CAD build for the part. Positions are in the model's coordinates, mm. Face numbers are marked on the shaded views. A direction names the side the tool comes from. Coordinates: 2 decimals unless noted, no trailing zeros. Order: outer loops, then holes, each group sorted by start corner. A loop starts at its lowest first (then second) coordinate and runs counter-clockwise, first axis right, second up. Notation, with made-up numbers: M 30.25,6 L 46.25,6 A28 ccw 46.25,37 Z; hole C -18.5,11 d5. An arc over 180 degrees is marked long. Write item = value, one per line.
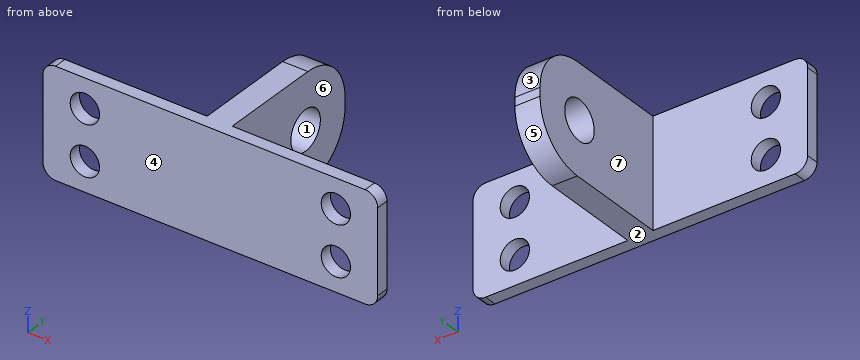
from build123d import *

# Parameters (mm, degrees)
SKETCH1_W           = 80
SKETCH1_H           = 26
SKETCH1_R           = 3.5
BOSS_EXTRUDE1_DEPTH = 3
FILLET1_R           = 2.9972
BOSS_EXTRUDE2_DEPTH = 36.322
FILLET2_R           = 11.9888
CUT_EXTRUDE1_REACH  = 45
SKETCH3_R           = 4.75


with BuildPart() as part:
    # Sketch1 → Boss-Extrude1 (new body)
    with BuildSketch(Plane(origin=(0, 0, 0), x_dir=(1, 0, 0), z_dir=(0, 1, 0))):
        with Locations((40, -13)):
            Rectangle(SKETCH1_W, SKETCH1_H)
        with Locations(Location((10, -19, 0), (0, 0, 270))):  # turned: the seam where the file's is
            Circle(SKETCH1_R, mode=Mode.SUBTRACT)
        with Locations(Location((10, -7, 0), (0, 0, 90))):  # turned: the seam where the file's is
            Circle(SKETCH1_R, mode=Mode.SUBTRACT)
        with Locations(Location((70, -7, 0), (0, 0, 270))):  # turned: the seam where the file's is
            Circle(SKETCH1_R, mode=Mode.SUBTRACT)
        with Locations(Location((70, -19, 0), (0, 0, 90))):  # turned: the seam where the file's is
            Circle(SKETCH1_R, mode=Mode.SUBTRACT)
    extrude(amount=BOSS_EXTRUDE1_DEPTH)

    # Fillet1
    fillet1_edges = [part.edges().sort_by_distance(p)[0] for p in [
        (0, 1.5, 0),
        (80, 1.5, 0),
        (80, 1.5, 26),
        (0, 1.5, 26),
    ]]
    fillet(fillet1_edges, radius=FILLET1_R)

    # Sketch2 → Boss-Extrude2 (add)
    with BuildSketch(Plane(origin=(0, 3, 0), x_dir=(1, 0, 0), z_dir=(0, 1, 0))):
        Polygon((43, 0), (40, 0), (37, 0), (37, -26), (40, -26), (43, -26), align=None)
    extrude(amount=BOSS_EXTRUDE2_DEPTH)

    # Fillet2
    fillet2_edges = [part.edges().sort_by_distance(p)[0] for p in [
        (40, 39.322, 26),
        (40, 39.322, 0),
    ]]
    fillet(fillet2_edges, radius=FILLET2_R)

    # Sketch3 → Cut-Extrude1 (cut, up to next)
    with BuildSketch(Plane.ZY.offset(-37), mode=Mode.PRIVATE) as cut_extrude1_sk1:
        with Locations((13, 26.622)):
            Circle(SKETCH3_R)
    cut_extrude1_tool1 = extrude(cut_extrude1_sk1.sketch, amount=-CUT_EXTRUDE1_REACH, mode=Mode.PRIVATE) & part.part
    add(cut_extrude1_tool1.solids().sort_by_distance((37, 26.622, 13))[0], mode=Mode.SUBTRACT)


solid = part.part
(1) Slice it at B-B, the plane z = 13. Write the cut outline in (x, y), then the cut area to 3 significant figures.
Evaluation:
outline = M 0,0 L 80,0 L 80,3 L 43,3 L 43,21.87 L 37,21.87 L 37,3 L 0,3 Z; M 37,31.37 L 43,31.37 L 43,39.32 L 37,39.32 Z
area = 401 mm²
(2) Slice it at C-C, the plane y = 23.5. Write the cut outline in (x, z).
Evaluation:
outline = M 37,0 L 43,0 L 43,9.42 L 37,9.42 Z; M 37,16.58 L 43,16.58 L 43,26 L 37,26 Z
(3) Wall check: line 1 (X direction, y = 1.2, z = 19); line 2 (Y direction, x = 41.65, z = 13); line 3 (X direction, y = 9, z = 17.5). Give the ranges that are in metal, low to high. Write a range as from..to.
Evaluation:
line_1 = 0..6.5, 13.5..66.5, 73.5..80
line_2 = 0..21.87, 31.37..39.32
line_3 = 37..43
(4) Tool access for the marked faces 5, 6 and 7: list every direction of +Z, -Z, +X, -X, +Y, -Y with a clear straight run to the whole face (end or side of a thin tool).
Evaluation:
face_5 = -Z, +X, -X, +Y
face_6 = +Z, -Z, +X, +Y
face_7 = +Z, -Z, -X, +Y
(5) Pull direction Z, two halves, no side cores. Call the marked faces 1, 2, 3 and 4: +Z half, -Z half, draft (parallel to the pull), parting line (faces both ways), or undercut.
Evaluation:
face_1 = undercut
face_2 = -Z half
face_3 = +Z half
face_4 = draft
(6) Slice it at A-A, the plane x = 10. Write the cut outline in (y, z).
Evaluation:
outline = M 0,0 L 3,0 L 3,3.5 L 0,3.5 Z; M 0,10.5 L 3,10.5 L 3,15.5 L 0,15.5 Z; M 0,22.5 L 3,22.5 L 3,26 L 0,26 Z
(7) Slice it at D-D, the plane z = 19. Write the cut outline in (x, y).
Evaluation:
outline = M 0,0 L 6.5,0 L 6.5,3 L 0,3 Z; M 13.5,0 L 66.5,0 L 66.5,3 L 43,3 L 43,38.23 L 37,38.23 L 37,3 L 13.5,3 Z; M 73.5,0 L 80,0 L 80,3 L 73.5,3 Z
(8) Pin check, flat tips, straight feed: pin 1 Ø10 at (y, z) = (19.5, 23) entering from +X; pin 2 Ø11 at (x, z) = (70, 7) entering from +Y; pin 3 Ø8 at (y, z) = (27, 15.5) entering from -X. Stop position of each tip, or through.
Evaluation:
pin_1 = 43
pin_2 = 3
pin_3 = 37
